Build history of the part. All positions in model axes, mm. A direction names the side the tool comes from. Round coordinates to 2 decimals unless told otherwise and drop trailing zeros. Order: outer loops, then holes, each group sorted by start corner. A loop starts at its lowest first (then second) coordinate and runs counter-clockwise, first axis right, second up. Notation, with made-up numbers: (53.5, -2) -> (96.5, -2) arc R17 cw to (96.5, 15) -> close; hole circle Ø11 at (-5.75, -12.5). An arc over 180 degrees is marked (long way). Answer as CSV lines item,"result". Start each with the question number.
```python
from build123d import *

# Parameters (mm, degrees)
BOX241_W                  = 0.5
BOX241_H                  = 1
BOX241_DEPTH              = 15
BOX241_ROLL_ANGLE         = 46
BOX242_W                  = 0.5
BOX242_H                  = 1
BOX242_DEPTH              = 15
BOX242_ROLL_ANGLE         = -46
BOX240_W                  = 0.5
BOX240_H                  = 1
BOX240_DEPTH              = 11
FUSION023_PLACEMENT_ANGLE = 45.9


with BuildPart() as cubo241:
    # Box241 → Box241 (new body)
    with BuildSketch(Plane.XY):
        with Locations((0.25, 0.5)):
            Rectangle(BOX241_W, BOX241_H)
    extrude(amount=BOX241_DEPTH)


with BuildPart() as cubo241_1:
    # Box241 roll: moved
    add(cubo241.part.rotate(Axis((0, 0, 0), (1, 0, 0)), BOX241_ROLL_ANGLE))


with BuildPart() as cubo241_2:
    # Box241 placement: moved
    add(cubo241_1.part.moved(Location((0, 11, 0.5))))


with BuildPart() as cubo242:
    # Box242 → Box242 (new body)
    with BuildSketch(Plane.XY):
        with Locations((0.25, 0.5)):
            Rectangle(BOX242_W, BOX242_H)
    extrude(amount=BOX242_DEPTH)


with BuildPart() as cubo242_1:
    # Box242 roll: moved
    add(cubo242.part.rotate(Axis((0, 0, 0), (1, 0, 0)), BOX242_ROLL_ANGLE))


with BuildPart() as cubo242_2:
    # Box242 placement: moved
    add(cubo242_1.part.moved(Location((0, 0.4, 1.1))))


with BuildPart() as fusion023:
    # Box240 → Box240 (new body)
    with BuildSketch(Plane.XY.offset(0.5)):
        with Locations((0.25, 0.5)):
            Rectangle(BOX240_W, BOX240_H)
    extrude(amount=BOX240_DEPTH)

    # Fusion023: union Cubo241, Cubo242
    add(cubo241_2.part)
    add(cubo242_2.part)


with BuildPart() as fusion023_1:
    # Fusion023 placement: moved
    add(fusion023.part.moved(Location((-171.4, 159.89, 0))).rotate(Axis((-171.4, 159.89, 0), (0, 0, -1)), FUSION023_PLACEMENT_ANGLE))


solid = fusion023_1.part
```
Q1. Which spindle directions (+Z, -Z, +X, -X, +Y, -Y) get a long thin tool onto all of the face, cutting with end or side? Do faces 1 (the face through (-164.53, 166.2, 8.33)), 2 (the face through (-171, 160, 0.5)), 3 (the face through (-171, 160, 11.5)), 4 (the face through (-167.07, 163.39, 6)). Say none if no direction does.
Q2. Slice it at C-C, the plane z = 8. Write the cut outline in (x, y).
Q3. Slice it at A-A, the plane y = 161.75. Write the cut outline in (x, z), plus the area to 3 significant figures.
Q4. Flat gauge pins, fed straight in: pin 1 Ø2 at (y, z) = (165.5, 8.5) entering from -X; pin 2 Ø1 at (x, z) = (-164, 10.5) entering from +Y; pin 3 Ø1 at (x, z) = (-167.5, 4) entering from +Y. Where does each tip first touch, or does it go through?
Q5. Two-plate mould, pull along Z, no slides. Class faces 5 (the face through (-163.08, 167.61, 0.86)), 6 (the face through (-168.956, 161.915, 3.769)), 7 (the face through (-168.68, 162.18, 9.09)): +Z half, -Z half, draft (parallel to the pull), parting line (faces both ways), or undercut.
Q6. Slice it at B-B, the plane z = 5.75. Write the cut outline in (x, y).
Q7. Slice it at D-D, the plane y = 164.5. Write the cut outline in (x, z), plus the area to 3 significant figures.
Q8. Probe L1, parallel to Z at x = -168, y = 163; L2, parallel to X at y = 162.25, z = 7.5; L3, parallel to X at y = 164.5, z = 5.5. List the from-to ranges inside material, lowest first.
Solutions:
1,face 1,"+X, +Y"
1,face 2,"-Z, -X, -Y"
1,face 3,"+Z, -X, -Y"
1,face 4,"+Z, -Z, +X, -Y"
2,outline,"(-171.4, 159.89) -> (-171.05, 159.53) -> (-170.33, 160.23) -> (-170.68, 160.59) -> close; (-169.08, 162.14) -> (-168.73, 161.78) -> (-167.7, 162.78) -> (-168.04, 163.14) -> close; (-165.98, 165.14) -> (-165.63, 164.78) -> (-164.6, 165.78) -> (-164.95, 166.14) -> close"
3,outline,"(-169.48, 1.9) -> (-168.76, 2.4) -> (-168.76, 3.79) -> (-169.48, 3.29) -> close; (-169.48, 8.54) -> (-168.76, 8.04) -> (-168.76, 9.43) -> (-169.48, 9.93) -> close"
3,area,"2.00 mm2"
4,pin 1,"stops at x = -166.21"
4,pin 2,"stops at y = 167.55"
4,pin 3,"stops at y = 163.62"
5,face 5,"-Z half"
5,face 6,"undercut"
5,face 7,"+Z half"
6,outline,"(-171.4, 159.89) -> (-171.05, 159.53) -> (-170.33, 160.23) -> (-170.68, 160.59) -> close; (-167.65, 163.52) -> (-167.31, 163.16) -> (-166.02, 164.4) -> (-166.37, 164.76) -> close"
7,outline,"(-166.64, 4.73) -> (-165.92, 4.23) -> (-165.92, 5.62) -> (-166.36, 5.92) -> (-165.92, 6.22) -> (-165.92, 7.61) -> (-166.64, 7.11) -> close"
7,area,"1.94 mm2"
8,L1,"z = 3.77 to 5.16, 6.67 to 8.06"
8,L2,"x = -168.46 to -168.25"
8,L3,"x = -166.64 to -165.92"
